Source: CAD feature listing. Evaluate the final solid. Frame: model axes, mm. Face numbers are marked on the shaded views. A direction names the side the tool comes from. Give positions to 0.01 mm unless a question says otherwise; leave off trailing zeros. Write each loop counter-clockwise with the first axis right and the second up, starting at its lowest first coordinate (ties: lowest second). Pieces come first, ordered by that corner, then holes. Notation, with made-up numbers: (19, 8.5) -> (73, 8.5) arc R25 ccw to (73, 20.5) -> close; hole circle Ø10 at (63, 11). An arc over 180 degrees is marked (long way). Write item = value, one per line.
Autodesk Inventor part; units mm, degrees
ref_plane "YZ Plane" through (0, 0, 0) normal (1, 0, 0) x (0, 1, 0)
ref_plane "XZ Plane" through (0, 0, 0) normal (0, 1, 0) x (-1, 0, 0)
ref_plane "XY Plane" through (0, 0, 0) normal (0, 0, 1) x (1, 0, 0)
sketch "Tube_Core_Skt" plane through (0, 0, 0) normal (0, 0, 1) x (1, 0, 0)
  circle A0 centre (0, 0) radius 16.025
  circle A1 centre (0, 0) radius 19.025
  dimension "d2" = 3
  dimension "d3" = 32.05
extrude "Tube_Core" add sketch "Tube_Core_Skt" along normal blind 15
sketch "Screw_Core_Skt" plane through (0, 0, 0) normal (0, 1, 0) x (-1, 0, 0)
  line L0 (-19.025, 0) -> (-19.025, 15)
  line L1 (19.025, 15) -> (-19.025, 15)
  line L2 (19.025, 0) -> (19.025, 15)
  line L3 (-19.025, 0) -> (19.025, 0)
  line L4 (0, 15) -> (-27.025, 15) construction
  line L5 (-27.025, 15) -> (-27.025, 10) construction
  line L6 (-27.025, 0) -> (0, 0) construction
  line L7 (0, 0) -> (0, 15) construction
  line L8 (-27.025, 15) -> (-33.175, 15) construction
  line L9 (-33.175, 15) -> (-33.175, 0) construction
  line L10 (-33.175, 0) -> (-27.025, 0) construction
  line L11 (-33.175, 10) -> (-27.025, 10) construction
  line L12 (-27.025, 10) -> (-27.025, 0) construction
  line L13 (-31.175, 0) -> (-31.175, 7.85)
  line L14 (-31.175, 7.85) -> (-29.025, 10)
  line L15 (-27.025, 10) -> (-27.025, 0)
  line L16 (-31.175, 0) -> (-27.025, 0)
  line L17 (-29.025, 10) -> (-27.025, 10)
  point P0 (0, 0)
  dimension "d11" = 10
  dimension "d12" = 8
  dimension "d13" = 6.15
  dimension "d14" = 2
  dimension "d15" = 2
  dimension "d16" = 45
revolve "Screw_Core" add sketch "Screw_Core_Skt" angle 360 about axis through (33.175, 0, 15) along (0, 0, -1) contours L13 L14 L17 L15 L16
sketch "Screw_Bridge_Skt" plane through (0, 0, 0) normal (0, 0, 1) x (1, 0, 0)
  circle A0 centre (0, 0) radius 19.025
  circle A1 centre (33.175, 0) radius 6.15
  circle A2 centre (0, 0) radius 19.025
  line L0 (17.2095, 8.1107) -> (28.5035, 4)
  line L1 (17.2095, -8.1107) -> (28.5035, -4)
  line L2 (0, 0) -> (33.175, 0) construction
  point P0 (35.15, 0)
  dimension "d25" = 4
  dimension "d26" = 20
extrude "Screw_Bridge" add sketch "Screw_Bridge_Skt" along normal blind 7.5 contours A0 L0 A1 L1
mirror "Screw_Copy" about plane through (0, 0, 0) normal (1, 0, 0) of "Screw_Bridge", "Screw_Core"
fillet "Fillet" radius 2 7 edges at (-19.025, 0, 15) (22.8565, -6.0553, 7.5) (22.8565, 6.0553, 7.5) (39.325, 0, 10) (-22.8565, -6.0553, 7.5) (-22.8565, 6.0553, 7.5) (-39.325, 0, 10)
equation "\"d2\" = tube_wall_width"
equation "\"d3\" = tube_diam + tube_tolerance"
equation "\"d4\" = tube_wall_height"
equation "\"d11\" = screw_height"
equation "\"d12\" = screw_spacing"
equation "\"d13\" = 0.5 * screw_head_diam + screw_wall_width"
equation "\"d14\" = 0.5 * screw_tolerance + 0.5 * screw_body_diam"
equation "\"d15\" = screw_wall_width"
equation "\"d25\" = 2 * screw_wall_width"
equation "\"d27\" = 0.75 * screw_height"
equation "\"d41\" = fillet"
equation "\"tube_diam\" = 31.8"
equation "\"screw_body_diam\" = 3"
equation "\"screw_head_diam\" = 8.3"
equation "\"screw_head_height\" = 3"
equation "\"screw_spacing\" = 8"
equation "\"screw_height\" = 10"
equation "\"tube_tolerance\" = 0.25"
equation "\"tube_wall_width\" = 3"
equation "\"tube_wall_height\" = 15"
equation "\"screw_wall_width\" = 2"
equation "\"fillet\" = 2"
equation "\"tube_base\" = 2"
equation "\"tube_base_height\" = 2"
equation "\"screw_tolerance\" = 1"
equation "\"screw_length\" = 12.7"
equation "\"wood_width\" = 15"
equation "\"block_height\" = 15"
equation "\"screw_head_ang\" = 71.666667deg"
equation "\"screw_head_m\" = 71.666667deg"
properties part number "Counter_Support"
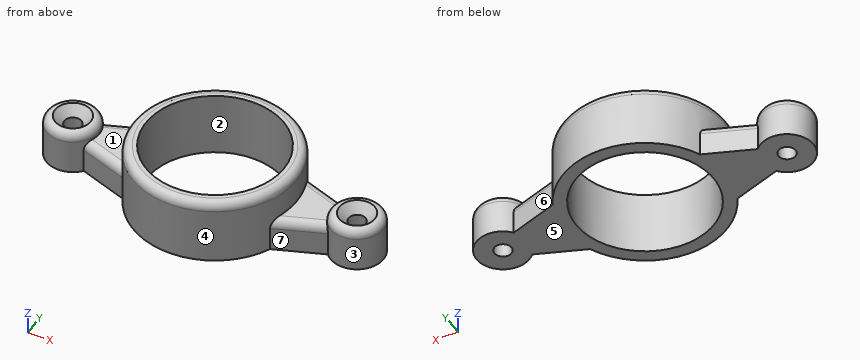
(1) Access query for the marked faces 4, 5, 6 and 7. Directions: +Z, -Z, +X, -X, +Y, -Y. A direction counts if a zero-diameter tool reaches every point of the face in a straight line with its end or side. Return the directions, or none.
Values follow:
face_4 = +Z
face_5 = -Z, +X, -X, +Y, -Y
face_6 = +Z, -Z, +Y
face_7 = +Z, -Z, -Y
(2) Pull-direction query (Y, two-part tool) for the marked faces 1, 2 and 3; classes: pulls with the +Y half, pulls with the -Y half, needs draft (parallel to the pull), parting line crosses it, or undercut.
Values follow:
face_1 = needs draft
face_2 = undercut
face_3 = parting line crosses it
(3) Section query D-D (z = 14). Return loops of the section in (x, y) (3 decimals).
Values follow:
outline = circle Ø37.515 at (0, 0); hole circle Ø32.05 at (0, 0)
(4) Section query B-B (y = 0). Give the number of separate pieces and of enclosed holes in the cut face, plus the area to 3 significant figures.
Values follow:
separate_pieces = 4
enclosed_holes = 0
area = 362 mm2
(5) Section query A-A (x = 0). Return loops of the section in (y, z) (1 decimal), plus the area to 3 significant figures.
Values follow:
outline = (-19, 0) -> (-16, 0) -> (-16, 15) -> (-17, 15) arc R2 ccw to (-19, 13) -> close; (16, 0) -> (19, 0) -> (19, 13) arc R2 ccw to (17, 15) -> (16, 15) -> close
area = 88.3 mm2
(6) First-contact query: pin 1 (2.5 mm diameter, centred on x = 34.5, y = -1, fed in from +Z); pin 2 (8 mm diameter, centred on y = 8.5, z = 11, fed in from +X); pin 3 (1.5 mm diameter, centred on x = 15.5, z = 9, fed in from -Y); pin 4 (2.5 mm diameter, centred on x = -33.175, y = 0, fed in from +Z). Flat tips, straight axial feed; report the tip coordinate or a pass-through.
Values follow:
pin_1 = 8.76
pin_2 = 36.22
pin_3 = -12.02
pin_4 = through
(7) Material intervals for line 1 (Y direction, x = 33, z = 4.5); line 2 (X direction, y = 1.5, z = 3); line 3 (Y direction, x = -7, z = 0.5), sorted ascending.
Values follow:
line_1 = -6.15 to -1.99, 1.99 to 6.15
line_2 = -39.14 to -34.5, -31.85 to -15.95, 15.95 to 31.85, 34.5 to 39.14
line_3 = -17.69 to -14.42, 14.42 to 17.69
